Autodesk Inventor part; units mm, degrees
ref_plane "YZ Plane" through (0, 0, 0) normal (1, 0, 0) x (0, 1, 0)
ref_plane "XZ Plane" through (0, 0, 0) normal (0, 1, 0) x (-1, 0, 0)
ref_plane "XY Plane" through (0, 0, 0) normal (0, 0, 1) x (1, 0, 0)
sketch "Sketch1" plane through (0, 0, 0) normal (0, 0, 1) x (1, 0, 0)
  line L0 (93.893, 28.1705) -> (89.575, 28.1705)
  line L1 (89.575, 12.9305) -> (89.575, 28.1705)
  line L2 (89.575, 7.8505) -> (89.575, 12.9305)
  line L3 (93.893, 7.8505) -> (89.575, 7.8505)
  line L4 (93.893, 7.8505) -> (93.893, 2.0085)
  line L5 (93.893, 2.0085) -> (96.433, 2.0085)
  line L6 (96.433, 7.8505) -> (96.433, 2.0085)
  line L7 (112.435, 7.8505) -> (96.433, 7.8505)
  line L8 (112.435, 7.8505) -> (112.435, 28.1705)
  line L9 (112.435, 28.1705) -> (96.433, 28.1705)
  line L10 (96.433, 34.0125) -> (96.433, 28.1705)
  line L11 (93.893, 34.0125) -> (96.433, 34.0125)
  line L12 (93.893, 34.0125) -> (93.893, 28.1705)
  line L13 (93.893, 6.5805) -> (89.575, 6.5805)
  line L14 (112.435, 6.5805) -> (96.433, 6.5805)
  line L15 (93.893, 29.4405) -> (89.575, 29.4405)
  line L16 (112.435, 29.4405) -> (96.433, 29.4405)
  line L17 (93.893, 6.5805) -> (93.643, 6.5805)
  line L18 (93.643, 6.5805) -> (93.643, 2.0085)
  line L19 (93.643, 2.0085) -> (93.643, 1.7585)
  line L20 (93.643, 1.7585) -> (90.143, 1.7585)
  line L21 (90.143, 1.7585) -> (90.143, 6.5805)
  line L22 (95.163, 2.0085) -> (95.163, 1.3114)
  line L23 (96.683, 6.5805) -> (96.683, 2.0085)
  line L24 (96.683, 2.0085) -> (96.683, 1.7585)
  line L25 (96.683, 1.7585) -> (100.183, 1.7585)
  line L26 (100.183, 1.7585) -> (100.183, 6.5805)
  line L27 (90.143, 1.7585) -> (100.183, 1.7585)
  line L28 (100.183, 1.7585) -> (100.183, -1.2415)
  line L29 (100.183, -1.2415) -> (90.143, -1.2415)
  line L30 (90.143, -1.2415) -> (90.143, 1.7585)
  line L31 (112.435, 18.0105) -> (108.4742, 18.0105)
  line L32 (93.893, 28.1705) -> (93.893, 34.0125)
  line L33 (93.893, 34.0125) -> (96.433, 34.0125)
  line L34 (96.433, 28.1705) -> (96.433, 34.0125)
  line L35 (112.435, 6.5805) -> (96.433, 6.5805)
  line L36 (93.643, 29.4405) -> (93.643, 34.0125)
  line L37 (93.643, 34.0125) -> (93.643, 34.2625)
  line L38 (93.643, 34.2625) -> (90.143, 34.2625)
  line L39 (90.143, 34.2625) -> (90.143, 29.4405)
  line L40 (95.163, 34.0125) -> (95.163, 34.7096)
  line L41 (96.683, 29.4405) -> (96.683, 34.0125)
  line L42 (100.183, 34.2625) -> (100.183, 29.4405)
  line L43 (96.683, 34.0125) -> (96.683, 34.2625)
  line L44 (96.683, 34.2625) -> (100.183, 34.2625)
  line L45 (90.143, 34.2625) -> (100.183, 34.2625)
  line L46 (100.183, 34.2625) -> (100.183, 37.2625)
  line L47 (100.183, 37.2625) -> (90.143, 37.2625)
  line L48 (90.143, 37.2625) -> (90.143, 34.2625)
  line L49 (96.683, 6.5805) -> (100.183, 6.5805)
  line L50 (100.183, 6.5805) -> (100.183, -1.2415)
  line L51 (100.183, -1.2415) -> (96.683, -1.2415)
  line L52 (96.683, -1.2415) -> (96.683, 6.5805)
  line L53 (96.683, 29.4405) -> (100.183, 29.4405)
  line L54 (100.183, 29.4405) -> (100.183, 37.2625)
  line L55 (100.183, 37.2625) -> (96.683, 37.2625)
  line L56 (96.683, 37.2625) -> (96.683, 29.4405)
  line L57 (90.143, 29.4405) -> (93.643, 29.4405)
  line L58 (93.643, 29.4405) -> (93.643, 37.2625)
  line L59 (93.643, 37.2625) -> (90.143, 37.2625)
  line L60 (90.143, 37.2625) -> (90.143, 29.4405)
  point P0 (0, 0)
  dimension "d0" = 0.25
  dimension "d1" = 0.25
  dimension "d2" = 3.5
  dimension "d3" = 3
extrude "Extrusion1" add sketch "Sketch1" along normal blind 12.7 contours L15 L39 L38 L37 L36 | L45 L58 L47 L56 | L48 L47 L58 L38 | L44 L42 L16 L41 L43 | L56 L47 L46 L44 | L18 L19 L20 L21 L13 | L27 L52 L29 L30 L20 | L24 L23 L14 L26 L25 | L25 L28 L29 L52
sketch "Sketch2" plane through (0, 0, 12.7) normal (0, 0, 1) x (1, 0, 0)
  line L0 (90.143, 6.5805) -> (90.143, -1.2415)
  line L1 (100.183, 29.4405) -> (100.183, 37.2625)
  line L2 (90.143, -1.2415) -> (100.183, -1.2415)
  line L3 (100.183, -1.2415) -> (100.183, 37.2625)
  line L4 (100.183, 37.2625) -> (90.143, 37.2625)
  line L5 (90.143, 37.2625) -> (90.143, -1.2415)
  point P0 (0, 0)
extrude "Extrusion2" add sketch "Sketch2" along normal blind 1
sketch "Sketch3" plane through (0, 0, 0) normal (0, 0, -1) x (-1, 0, 0)
  line L0 (-90.143, -1.2415) -> (-100.183, -1.2415)
  line L1 (-100.183, 37.2625) -> (-90.143, 37.2625)
  line L2 (-90.143, -1.2415) -> (-100.183, -1.2415)
  line L3 (-100.183, -1.2415) -> (-100.183, -7.5915)
  line L4 (-100.183, -7.5915) -> (-90.143, -7.5915)
  line L5 (-90.143, -7.5915) -> (-90.143, -1.2415)
  line L6 (-100.183, 29.4405) -> (-100.183, 37.2625)
  line L7 (-100.183, 37.2625) -> (-90.143, 37.2625)
  line L8 (-90.143, 37.2625) -> (-90.143, 43.6125)
  line L9 (-90.143, 43.6125) -> (-100.183, 43.6125)
  line L10 (-100.183, 43.6125) -> (-100.183, 37.2625)
  circle A0 centre (-95.163, -4.4165) radius 1.25
  circle A1 centre (-95.163, 40.4375) radius 1.25
  point P0 (0, 0)
  point P1 (-90.143, -4.4165)
  point P2 (-90.143, 40.4375)
  point P3 (-95.163, 43.6125)
  point P4 (-95.163, -7.5915)
  dimension "d8" = 6.35
  dimension "d9" = 6.35
  dimension "d10" = 2.5
  dimension "d11" = 2.5
extrude "Extrusion3" add sketch "Sketch3" against normal blind 1
fillet "Fillet2" radius 1 4 edges at (90.143, 43.6125, 0.5) (100.183, 43.6125, 0.5) (90.143, -7.5915, 0.5) (100.183, -7.5915, 0.5)
sketch "Sketch4" plane through (0, 0, 0) normal (0, 0, -1) x (-1, 0, 0)
  line L0 (-100.183, 6.5805) -> (-96.683, 6.5805)
  line L1 (-96.683, 6.5805) -> (-96.683, 5.5805)
  line L2 (-96.683, 6.5805) -> (-96.683, 1.7585)
  line L3 (-96.683, 5.5805) -> (-100.1874, 5.5805)
  line L4 (-100.1874, 5.5805) -> (-100.1874, 6.5805)
  line L5 (-100.1874, 6.5805) -> (-96.683, 6.5805)
  line L6 (-94.143, 2.0085) -> (-94.143, 7.8505)
  line L7 (-94.143, 6.5805) -> (-89.825, 6.5805)
  line L8 (-90.143, 29.4405) -> (-90.143, 6.5805)
  line L9 (-94.143, 5.5805) -> (-90.143, 5.5805)
  line L10 (-90.143, 5.5805) -> (-90.143, 6.5805)
  line L11 (-90.143, 6.5805) -> (-94.143, 6.5805)
  line L12 (-94.143, 6.5805) -> (-94.143, 5.5805)
  line L13 (-100.183, 6.5805) -> (-100.183, 29.4405)
  line L14 (-100.183, 18.0105) -> (-103.7607, 18.0105)
  line L15 (-100.183, 29.4405) -> (-96.683, 29.4405)
  line L16 (-96.683, 29.4405) -> (-96.683, 30.4405)
  line L17 (-96.683, 29.4405) -> (-96.683, 34.2625)
  line L18 (-96.683, 30.4405) -> (-100.1874, 30.4405)
  line L19 (-100.1874, 30.4405) -> (-100.1874, 29.4405)
  line L20 (-100.1874, 29.4405) -> (-96.683, 29.4405)
  line L21 (-94.143, 34.0125) -> (-94.143, 28.1705)
  line L22 (-94.143, 29.4405) -> (-89.825, 29.4405)
  line L23 (-90.143, 6.5805) -> (-90.143, 29.4405)
  line L24 (-94.143, 30.4405) -> (-90.143, 30.4405)
  line L25 (-90.143, 30.4405) -> (-90.143, 29.4405)
  line L26 (-90.143, 29.4405) -> (-94.143, 29.4405)
  line L27 (-94.143, 29.4405) -> (-94.143, 30.4405)
  line L28 (-100.183, 29.4405) -> (-100.183, 6.5805)
  point P0 (0, 0)
  dimension "d17" = 1
  dimension "d23" = 1
extrude "Extrusion4" cut sketch "Sketch4" against normal up to surface (12.7 mm away)
fillet "Fillet4" radius 1 8 edges at (96.683, 5.5805, 6.35) (100.183, 5.5805, 6.35) (93.643, 5.5805, 6.35) (90.143, 5.5805, 6.35) (100.183, 30.4405, 6.35) (96.683, 30.4405, 6.35) (93.643, 30.4405, 6.35) (90.143, 30.4405, 6.35)
fillet "Fillet5" radius 1 4 edges at (100.183, -1.2415, 7.35) (90.143, -1.2415, 7.35) (100.183, 37.2625, 7.35) (90.143, 37.2625, 7.35)
fillet "Fillet6" radius 1 8 edges at (90.4359, -0.9486, 13.7) (95.163, -1.2415, 13.7) (99.8901, -0.9486, 13.7) (100.183, 18.0105, 13.7) (99.8901, 36.9696, 13.7) (95.163, 37.2625, 13.7) (90.4359, 36.9696, 13.7) (90.143, 18.0105, 13.7)
sketch "Sketch5" plane through (0, 0, 0) normal (0, 0, -1) x (-1, 0, 0)
  line L0 (-96.683, 1.7585) -> (-93.643, 1.7585)
  line L1 (-96.683, 1.7585) -> (-93.643, 1.7585)
  line L2 (-93.643, 1.7585) -> (-93.643, 1.2585)
  line L3 (-93.643, 1.2585) -> (-96.683, 1.2585)
  line L4 (-96.683, 1.2585) -> (-96.683, 1.7585)
  line L5 (-100.183, 4.5805) -> (-100.183, 31.4405)
  line L6 (-100.183, 18.0105) -> (-106.4704, 18.0105)
  line L7 (-96.683, 34.2625) -> (-93.643, 34.2625)
  line L8 (-96.683, 34.2625) -> (-93.643, 34.2625)
  line L9 (-93.643, 34.2625) -> (-93.643, 34.7625)
  line L10 (-93.643, 34.7625) -> (-96.683, 34.7625)
  line L11 (-96.683, 34.7625) -> (-96.683, 34.2625)
  point P0 (0, 0)
  dimension "d24" = 0.5
extrude "Extrusion5" cut sketch "Sketch5" against normal up to surface (12.7 mm away)
properties part number "BackWheelServoClasp"
Check sheet for the modelled part. Datum: model origin and axes. Units: mm. A direction names the side the tool comes from. Round coordinates to 2 decimals unless told otherwise and drop trailing zeros. Write each loop counter-clockwise with the first axis right and the second up, starting at its lowest first coordinate (ties: lowest second). Pieces come first, ordered by that corner, then holes. Notation, with made-up numbers: (10, -37) - (65, -37) arc R15 cw to (65, -18) - close; hole circle Ø10 at (25, 84.5). An arc over 180 degrees is marked (long way). Return JSON: item names as keys, results as strings.
Q1. Draft check along Y on faces 1 (the flat face through (95, -1, 0)), 2 (the cylindrical face through (90.43, 30.74, 6.44)), 3 (the cylindrical face through (99.9, 43.31, 0.51)). Enter one of: released by +Y, released by -Y, zero draft, split by the parting line, or undercut.
Returned:
{"face 1": "zero draft", "face 2": "undercut", "face 3": "released by +Y"}
Q2. Cross-section at A-A (z = 9.25). Record the boundary of the cut face in (x, y), then the cut area to 3 significant figures.
Returned:
{"outline": "(90.14, -0.24) arc R1 ccw to (91.14, -1.24) - (99.18, -1.24) arc R1 ccw to (100.18, -0.24) - (100.18, 4.58) arc R1 ccw to (99.18, 5.58) - (97.68, 5.58) arc R1 ccw to (96.68, 4.58) - (96.68, 1.26) - (93.64, 1.26) - (93.64, 4.58) arc R1 ccw to (92.64, 5.58) - (91.14, 5.58) arc R1 ccw to (90.14, 4.58) - close; (90.14, 31.44) arc R1 ccw to (91.14, 30.44) - (92.64, 30.44) arc R1 ccw to (93.64, 31.44) - (93.64, 34.76) - (96.68, 34.76) - (96.68, 31.44) arc R1 ccw to (97.68, 30.44) - (99.18, 30.44) arc R1 ccw to (100.18, 31.44) - (100.18, 36.26) arc R1 ccw to (99.18, 37.26) - (91.14, 37.26) arc R1 ccw to (90.14, 36.26) - close", "area": "108 mm²"}
Q3. Access from +Z, -Z, +X, -X, +Y, -Y to the whole of each face (thin tool, end or side, straight path). Record for faces 4 (the cylindrical face through (99.88, 5.3, 6.26)), 5 (the cylindrical face through (90.444, 5.295, 6.439)), 6 (the flat face through (96.683, 33, 6)), 7 (the cylindrical face through (99.88, 36.98, 6.77)), 8 (the flat face through (98, 30.44, 6)).
Returned:
{"face 4": "-Z, +X", "face 5": "-Z, -X", "face 6": "-Z", "face 7": "+Z, +X, +Y", "face 8": "-Z, +X, -X"}
Q4. Cross-section at D-D (y = -2.5). Record the boundary of the cut face in (x, z).
Returned:
{"outline": "(90.14, 0) - (100.18, 0) - (100.18, 1) - (90.14, 1) - close"}
Q5. Depth check by flat-ended pin: P1, Ø3, axis at x = 92, y = 16.5, coming from the -Z side; P2, Ø3.5, axis at x = 95, z = 4.5, coming from the +Y side; P3, Ø2, axis at x = 94.5, y = -3.5, coming from the +Z side; P4, Ø5, axis at y = 25, z = 12, coming from the +X side. Enter the tip coordinate at first touch or a pass-through.
Returned:
{"P1": "stops at z = 12.7", "P2": "stops at y = 37.26", "P3": "stops at z = 1", "P4": "stops at x = 100.18"}
Q6. Scan lines: L1, parallel to Y at x = 99.25, z = 6.75; L2, parallel to Y at x = 91, z = 5.5; L3, parallel to Z at x = 94.75, y = 22.5. Record each from-to range of solid material in increasing order. Write a range as from..to.
Returned:
{"L1": "y = -1.24..5.58, 30.44..37.26", "L2": "y = -1.23..5.57, 30.45..37.25", "L3": "z = 12.7..13.7"}
Q7. Cross-section at B-B (y = 33.5). Record the boundary of the cut face in (x, z).
Returned:
{"outline": "(90.14, 0) - (93.64, 0) - (93.64, 12.7) - (96.68, 12.7) - (96.68, 0) - (100.18, 0) - (100.18, 12.7) arc R1 ccw to (99.18, 13.7) - (91.14, 13.7) arc R1 ccw to (90.14, 12.7) - close"}
